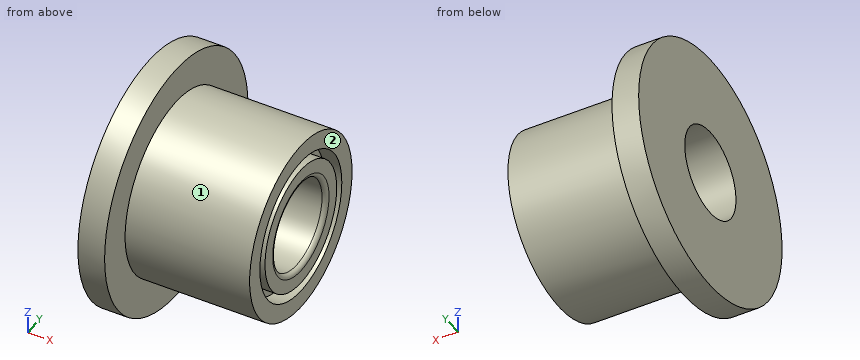
Autodesk Inventor part; units mm, degrees
ref_plane "YZ Plane" through (0, 0, 0) normal (1, 0, 0) x (0, 1, 0)
ref_plane "XZ Plane" through (0, 0, 0) normal (0, 1, 0) x (-1, 0, 0)
ref_plane "XY Plane" through (0, 0, 0) normal (0, 0, 1) x (1, 0, 0)
sketch "スケッチ1" plane through (0, 0, 0) normal (1, 0, 0) x (0, 1, 0)
  circle A0 centre (0, 0) radius 5
  circle A1 centre (0, 0) radius 10
  circle A2 centre (0, 0) radius 8
  circle A3 centre (0, 0) radius 7
  circle A4 centre (0, 0) radius 14
  dimension "d0" = 10
  dimension "d1" = 20
  dimension "d2" = 2
  dimension "d8" = 2
  dimension "d9" = 28
extrude "押し出し1" add sketch "スケッチ1" along normal blind 17 contours A1 | A3
extrude "押し出し2" add sketch "スケッチ1" along normal blind 15 contours A2
fillet "フィレット1" radius 0.5 1 edges at (17, -5, 0)
extrude "押し出し3" add sketch "スケッチ1" along normal blind 3 contours A4
properties part number "myPartbasic"
Source: CAD feature listing. Evaluate the final solid. Frame: model axes, mm. Face numbers are marked on the shaded views. A direction names the side the tool comes from. Round coordinates to 2 decimals unless told otherwise and drop trailing zeros. Order: outer loops, then holes, each group sorted by start corner. A loop starts at its lowest first (then second) coordinate and runs counter-clockwise, first axis right, second up. Notation, with made-up numbers: (54, 17) - (70, 17) arc R28 cw to (70, 39) - close; hole circle Ø5 at (58.5, 46). An arc over 180 degrees is marked (long way). Use a Markdown table: item, result. Add a question column.
1. Line query: probe 1 along Z at (x, y) = (10.75, 0); probe 2 along Y at (x, z) = (15.75, -5.5); probe 3 along Y at (x, z) = (15.5, 6.25). Output: solid intervals per line, ascending.
2. Section query A-A (y = 0). Return the cut outline in (x, z), then the cut area to 3 significant figures.
3. Section query C-C (x = 9). Return the cut outline in (y, z), then the cut area to 3 significant figures.
4. First-contact query: pin 1 (2 mm diameter, centred on x = 10, z = 0, fed in from +Y); pin 2 (10 mm diameter, centred on x = 5, y = -5.5, fed in from -Z); pin 3 (1.5 mm diameter, centred on x = 10.5, z = -2, fed in from -Y); pin 4 (5 mm diameter, centred on y = -6.5, z = -7, fed in from -X). Flat tips, straight axial feed; report the tip coordinate or a pass-through.
5. Section query D-D (z = 6). Return the cut outline in (x, y).
6. Set-up query: the marked faces 1 and 2. Return all of +Z, -Z, +X, -X, +Y, -Y with unobstructed straight access to the full face (end or side cutting, diameter ignored); none if empty.
Derived:
| question | item | result |
|---|---|---|
| 1 | probe 1 | -10 to -5, 5 to 10 |
| 1 | probe 2 | -8.35 to -5.81, -4.33 to 4.33, 5.81 to 8.35 |
| 1 | probe 3 | -7.81 to -4.99, -3.15 to 3.15, 4.99 to 7.81 |
| 2 | outline | (0, -14) - (3, -14) - (3, -10) - (17, -10) - (17, -8) - (15, -8) - (15, -7) - (17, -7) - (17, -5.5) arc R0.5 ccw to (16.5, -5) - (0, -5) - close; (0, 5) - (16.5, 5) arc R0.5 ccw to (17, 5.5) - (17, 7) - (15, 7) - (15, 8) - (17, 8) - (17, 10) - (3, 10) - (3, 14) - (0, 14) - close |
| 2 | area | 190 mm2 |
| 3 | outline | circle Ø20 at (0, 0); hole circle Ø10 at (0, 0) |
| 3 | area | 236 mm2 |
| 4 | pin 1 | y = 10 |
| 4 | pin 2 | z = -13.97 |
| 4 | pin 3 | y = -9.92 |
| 4 | pin 4 | x = 0 |
| 5 | outline | (0, -12.65) - (3, -12.65) - (3, -8) - (17, -8) - (17, -5.29) - (15, -5.29) - (15, -3.61) - (17, -3.61) - (17, 3.61) - (15, 3.61) - (15, 5.29) - (17, 5.29) - (17, 8) - (3, 8) - (3, 12.65) - (0, 12.65) - close |
| 6 | face 1 | +X |
| 6 | face 2 | +Z, -Z, +X, +Y, -Y |
